```python
from build123d import *

# Parameters (mm, degrees)
SKETCH1_R           = 20.75
BOSS_EXTRUDE1_DEPTH = 6.5
CUT_EXTRUDE1_START  = -1
SKETCH2_R           = 20.75
SKETCH2_R_2         = 19.75
CUT_EXTRUDE1_DEPTH  = 1
CUT_EXTRUDE2_START  = -1.5
SKETCH3_R           = 20.75
SKETCH3_R_2         = 19.75
CUT_EXTRUDE2_DEPTH  = 1.5
CHAMFER1_SIZE       = 1.5
SKETCH4_R           = 18.75
CUT_EXTRUDE3_DEPTH  = 4.5
CUT_EXTRUDE4_DEPTH  = 3.5
CIRPATTERN1_COUNT   = 8
SKETCH6_R           = 5.5
SKETCH6_R_2         = 1.5
CUT_EXTRUDE5_DEPTH  = 3.5


with BuildPart() as part:
    # Sketch1 → Boss-Extrude1 (new body)
    with BuildSketch(Plane(origin=(0, 0, 0), x_dir=(1, 0, 0), z_dir=(0, 1, 0))):
        with Locations(Location((0, 0, 0), (0, 0, 90))):
            Circle(SKETCH1_R)
    extrude(amount=BOSS_EXTRUDE1_DEPTH)

    # Sketch2 → Cut-Extrude1 (cut)
    with BuildSketch(Plane(origin=(0, 5.5, 0), x_dir=(1, 0, 0), z_dir=(0, 1, 0)).offset(CUT_EXTRUDE1_START)):
        with Locations(Location((0, 0, 0), (0, 0, 90))):
            Circle(SKETCH2_R)
        with Locations(Location((0, 0, 0), (0, 0, 270))):
            Circle(SKETCH2_R_2, mode=Mode.SUBTRACT)
    extrude(amount=CUT_EXTRUDE1_DEPTH, mode=Mode.SUBTRACT)

    # Sketch3 → Cut-Extrude2 (cut)
    with BuildSketch(Plane(origin=(0, 3.5, 0), x_dir=(1, 0, 0), z_dir=(0, 1, 0)).offset(CUT_EXTRUDE2_START)):
        with Locations(Location((0, 0, 0), (0, 0, 90))):
            Circle(SKETCH3_R)
        with Locations(Location((0, 0, 0), (0, 0, 270))):
            Circle(SKETCH3_R_2, mode=Mode.SUBTRACT)
    extrude(amount=CUT_EXTRUDE2_DEPTH, mode=Mode.SUBTRACT)

    # Chamfer1
    chamfer1_edges = [part.edges().sort_by_distance(p)[0] for p in [
        (0, 0, 20.75),
    ]]
    chamfer(chamfer1_edges, length=CHAMFER1_SIZE)

    # Sketch4 → Cut-Extrude3 (cut)
    with BuildSketch(Plane(origin=(0, 6.5, 0), x_dir=(1, 0, 0), z_dir=(0, 1, 0))):
        with Locations(Location((0, 0, 0), (0, 0, 270))):
            Circle(SKETCH4_R)
    extrude(amount=-CUT_EXTRUDE3_DEPTH, mode=Mode.SUBTRACT)

    # Sketch5 → Cut-Extrude4 (cut)
    with BuildSketch(Plane.XZ):
        with BuildLine():
            ThreePointArc((6, -20.75), (0, -17.750879894), (-6, -20.75))
            ThreePointArc((-6, -20.75), (0, -23.235281374), (6, -20.75))
        make_face()
    cut_extrude4 = extrude(amount=-CUT_EXTRUDE4_DEPTH, mode=Mode.SUBTRACT)

    # CirPattern1: Cut-Extrude4 ×8 about axis
    cirpattern1_axis = Axis((0, 0, 0), (0, 1, 0))
    for i in range(1, CIRPATTERN1_COUNT):
        add(cut_extrude4.rotate(cirpattern1_axis, i * 360 / CIRPATTERN1_COUNT), mode=Mode.SUBTRACT)

    # Sketch6 → Cut-Extrude5 (cut)
    with BuildSketch(Plane(origin=(0, 0, 0), x_dir=(-1, 0, 0), z_dir=(0, -1, 0))):
        with Locations(Location((0, 0, 0), (0, 0, 90))):
            Circle(SKETCH6_R)
        with BuildLine():
            ThreePointArc((3.786151182, 8.164867374), (2.083317107, 12.812485701), (6.730935434, 14.515319775))
            ThreePointArc((6.730935434, 14.515319775), (10.993885508, 11.624735757), (14.117584779, 7.529528538))
            ThreePointArc((14.117584779, 7.529528538), (12.676447476, 2.7942225), (7.941141438, 4.235359803))
            ThreePointArc((7.941141438, 4.235359803), (6.184060598, 6.538913863), (3.786151182, 8.164867374))
        make_face()
        with Locations(Location((0, 9.5, 0), (0, 0, 90))):
            Circle(SKETCH6_R_2)
        with BuildLine():
            ThreePointArc((-6.730935434, 14.515319775), (-10.993885508, 11.624735757), (-14.117584779, 7.529528538))
            ThreePointArc((-14.117584779, 7.529528538), (-12.676447476, 2.7942225), (-7.941141438, 4.235359803))
            ThreePointArc((-7.941141438, 4.235359803), (-6.184060598, 6.538913863), (-3.786151182, 8.164867374))
            ThreePointArc((-3.786151182, 8.164867374), (-2.083317107, 12.812485701), (-6.730935434, 14.515319775))
        make_face()
        with Locations(Location((-12.5, 0, 0), (0, 0, 90))):
            Circle(SKETCH6_R_2)
        with BuildLine():
            ThreePointArc((-3.786151182, -8.164867374), (-2.083317107, -12.812485701), (-6.730935434, -14.515319775))
            ThreePointArc((-6.730935434, -14.515319775), (-10.993885508, -11.624735757), (-14.117584779, -7.529528538))
            ThreePointArc((-14.117584779, -7.529528538), (-12.676447476, -2.7942225), (-7.941141438, -4.235359803))
            ThreePointArc((-7.941141438, -4.235359803), (-6.184060598, -6.538913863), (-3.786151182, -8.164867374))
        make_face()
        with BuildLine():
            ThreePointArc((6.730935434, -14.515319775), (10.993885508, -11.624735757), (14.117584779, -7.529528538))
            ThreePointArc((14.117584779, -7.529528538), (12.676447476, -2.7942225), (7.941141438, -4.235359803))
            ThreePointArc((7.941141438, -4.235359803), (6.184060598, -6.538913863), (3.786151182, -8.164867374))
            ThreePointArc((3.786151182, -8.164867374), (2.083317107, -12.812485701), (6.730935434, -14.515319775))
        make_face()
        with Locations(Location((12.5, 0, 0), (0, 0, 90))):
            Circle(SKETCH6_R_2)
        with Locations(Location((0, -9.5, 0), (0, 0, 90))):
            Circle(SKETCH6_R_2)
    extrude(amount=-CUT_EXTRUDE5_DEPTH, mode=Mode.SUBTRACT)


solid = part.part
```
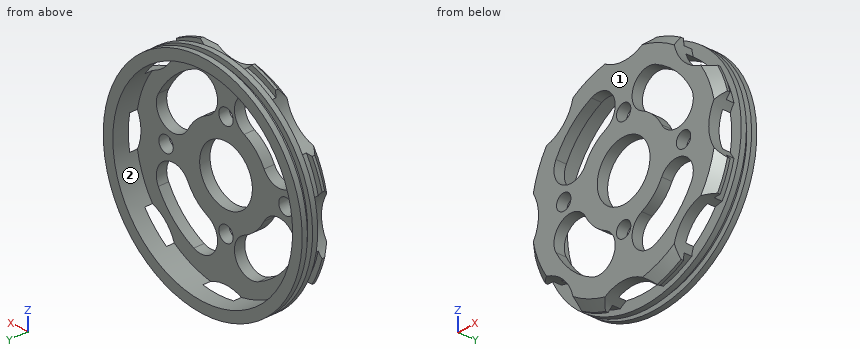
Source: CAD feature listing. Evaluate the final solid. Frame: model axes, mm. Face numbers are marked on the shaded views. Round coordinates to 2 decimals unless told otherwise and drop trailing zeros. Use CSV: the item, a comma, the result in double quotes. Start each with the question number.
Q1. First-contact query: P1, Ø6, axis at x = 1, z = -3.5, coming from the +Y side; P2, Ø1, axis at x = 15.5, y = 1.5, coming from the -Z side. Flat tips, straight axial feed; report the tip coordinate or a pass-through.
Q2. Cut plane A-A on z = 0. Count the separate pieces of the cut face and the enclosed holes in it, plus the area to 3 significant figures.
Q3. Pull-direction query (Z, two-part tool) for the marked faces 1 and 2; classes: +Z half, -Z half, draft (parallel to the pull), parting line (faces both ways), or undercut.
Q4. Line query: line 1 (X direction, y = 0.8, z = 0); line 2 (Z direction, x = -6, y = 1.75); line 3 (Z direction, x = 0.5, y = 5). Output: solid intervals per line, ascending. Write a range as from..to.
Results found:
1,P1,"y = 2"
1,P2,"z = -10.92"
2,separate pieces,"6"
2,enclosed holes,"0"
2,area,"47.0 mm^2"
3,face 1,"draft"
3,face 2,"undercut"
4,line 1,"-17.75..-14, -11..-5.5, 5.5..11, 14..17.75"
4,line 2,"-19.86..-14.76, -6.71..6.71, 14.76..19.86"
4,line 3,"-19.74..-18.74, 18.74..19.74"
